Design review of the part built by this model. Coordinates are the model's own, in mm. Give positions to 0.01 mm unless a question says otherwise; leave off trailing zeros. Order: outer loops, then holes, each group sorted by start corner. A loop starts at its lowest first (then second) coordinate and runs counter-clockwise, first axis right, second up. Notation, with made-up numbers: M -17.5,-8 L 6.5,-8 A9 cw 6.5,5 Z; hole C 79.25,19 d7. An arc over 180 degrees is marked long. Answer as a JSON object with one key per item and string values.
from build123d import *

# Parameters (mm, degrees)
SKETCH1_W           = 111.7
SKETCH1_H           = 112
SKETCH1_R           = 1.65
SKETCH1_R_2         = 1.875
BOSS_EXTRUDE1_DEPTH = 1.6
FILLET1_R           = 4


with BuildPart() as part:
    # Sketch1 → Boss-Extrude1 (new body)
    with BuildSketch(Plane(origin=(0, 0, 0), x_dir=(1, 0, 0), z_dir=(0, 1, 0))):
        Rectangle(SKETCH1_W, SKETCH1_H)
        with Locations((-50.575, 50.725)):
            Circle(SKETCH1_R, mode=Mode.SUBTRACT)
        with Locations((-50.575, -50.725)):
            Circle(SKETCH1_R, mode=Mode.SUBTRACT)
        with Locations((50.575, 50.725)):
            Circle(SKETCH1_R, mode=Mode.SUBTRACT)
        with Locations((50.575, -50.725)):
            Circle(SKETCH1_R, mode=Mode.SUBTRACT)
        with Locations((26.45, -10.82)):
            Circle(SKETCH1_R_2, mode=Mode.SUBTRACT)
        with Locations((42.45, -10.82)):
            Circle(SKETCH1_R_2, mode=Mode.SUBTRACT)
        with Locations((42.45, 37.51)):
            Circle(SKETCH1_R_2, mode=Mode.SUBTRACT)
        with Locations((26.45, 37.51)):
            Circle(SKETCH1_R_2, mode=Mode.SUBTRACT)
        with Locations((-42.45, -10.82)):
            Circle(SKETCH1_R_2, mode=Mode.SUBTRACT)
        with Locations((-26.45, -10.82)):
            Circle(SKETCH1_R_2, mode=Mode.SUBTRACT)
        with Locations((-42.45, 37.51)):
            Circle(SKETCH1_R_2, mode=Mode.SUBTRACT)
        with Locations((-26.45, 37.51)):
            Circle(SKETCH1_R_2, mode=Mode.SUBTRACT)
    extrude(amount=BOSS_EXTRUDE1_DEPTH)

    # Fillet1
    fillet1_edges = [part.edges().sort_by_distance(p)[0] for p in [
        (55.85, 0.8, 56),
        (-55.85, 0.8, 56),
        (-55.85, 0.8, -56),
        (55.85, 0.8, -56),
    ]]
    fillet(fillet1_edges, radius=FILLET1_R)


solid = part.part
(1) To check wall thickness, follow L1, parallel to X at y = 0.7, z = -37.51 (3 decimals); L2, parallel to Z at x = 26.45, y = 0.5 (3 decimals); L3, parallel to X at y = 0.4, z = 50. State the ranges of each line that lie inside material, in increasing order. Write a range as from..to.
Checked values:
{"L1": "x = -55.85..-44.325, -40.575..-28.325, -24.575..24.575, 28.325..40.575, 44.325..55.85", "L2": "z = -56..-39.385, -35.635..8.945, 12.695..56", "L3": "x = -55.85..-52.06, -49.09..49.09, 52.06..55.85"}
(2) We need section B-B (z = -37.51). Write out the cut boundary in (x, y) (3 decimals).
Checked values:
{"outline": "M -55.85,0 L -44.325,0 L -44.325,1.6 L -55.85,1.6 Z; M -40.575,0 L -28.325,0 L -28.325,1.6 L -40.575,1.6 Z; M -24.575,0 L 24.575,0 L 24.575,1.6 L -24.575,1.6 Z; M 28.325,0 L 40.575,0 L 40.575,1.6 L 28.325,1.6 Z; M 44.325,0 L 55.85,0 L 55.85,1.6 L 44.325,1.6 Z"}
(3) Insertion check: pin 1 (3.5 mm diameter, centred on x = -42.45, z = -37.51, fed in from -Y). The pin has a flat end and moves straight along its axis. Give the tip position at first contact, or say it passes through.
Checked values:
{"pin 1": "passes through"}
(4) We need section A-A (x = 26.45). Write out the cut boundary in (y, z) (3 decimals), plus the area to 3 significant figures.
Checked values:
{"outline": "M 0,-56 L 1.6,-56 L 1.6,-39.385 L 0,-39.385 Z; M 0,-35.635 L 1.6,-35.635 L 1.6,8.945 L 0,8.945 Z; M 0,12.695 L 1.6,12.695 L 1.6,56 L 0,56 Z", "area": "167 mm^2"}
(5) Draft analysis for pull direction Z (two halves, no side actions). For faces 1 (the cylindrical face through (-28.323, 0.789, 10.738)), 2 (the cylindrical face through (54.647, 0.811, -54.859)), 3 (the flat face through (-1, 1.6, -1)), 4 (the cylindrical face through (-54.709, 0.811, 54.797)), state which applies: +Z half, -Z half, draft (parallel to the pull), parting line (faces both ways), or undercut.
Checked values:
{"face 1": "undercut", "face 2": "-Z half", "face 3": "draft", "face 4": "+Z half"}
